```python
from build123d import *

# Parameters (mm, degrees)
F0_R     = 2.4
F1_DEPTH = 3.93
F2_R     = 3.705


with BuildPart() as f1:
    # F0 (on Top) → F1 (new body)
    with BuildSketch(Plane.XY):
        with BuildLine():
            Line((-7.319459, -8.152287), (-7.319459, 4.142713))
            ThreePointArc((-7.319459, 4.142713), (-11.024459, 7.847713), (-14.729459, 4.142713))
            Line((-14.729459, 4.142713), (-14.729459, -15.562287))
            Line((-14.729459, -15.562287), (4.975541, -15.562287))
            ThreePointArc((4.975541, -15.562287), (8.680541, -11.857287), (4.975541, -8.152287))
            Line((4.975541, -8.152287), (-7.319459, -8.152287))
        make_face()
        with BuildLine():
            ThreePointArc((-8.624459, -11.857287), (-8.662221, -12.281351), (-8.774317, -12.69207))
            ThreePointArc((-8.774317, -12.69207), (-8.810969, -12.739379), (-8.868073, -12.757287))
            Line((-8.868073, -12.757287), (-9.624459, -12.757287))
            ThreePointArc((-9.624459, -12.757287), (-9.978012, -12.903734), (-10.124459, -13.257287))
            Line((-10.124459, -13.257287), (-10.124459, -14.013673))
            ThreePointArc((-10.124459, -14.013673), (-10.142367, -14.070777), (-10.189676, -14.107429))
            ThreePointArc((-10.189676, -14.107429), (-11.024459, -14.257287), (-11.859241, -14.107429))
            ThreePointArc((-11.859241, -14.107429), (-11.906551, -14.070777), (-11.924459, -14.013673))
            Line((-11.924459, -14.013673), (-11.924459, -13.257287))
            ThreePointArc((-11.924459, -13.257287), (-12.070905, -12.903734), (-12.424459, -12.757287))
            Line((-12.424459, -12.757287), (-13.180845, -12.757287))
            ThreePointArc((-13.180845, -12.757287), (-13.237949, -12.739379), (-13.274601, -12.69207))
            ThreePointArc((-13.274601, -12.69207), (-13.386697, -12.281351), (-13.424459, -11.857287))
            ThreePointArc((-13.424459, -11.857287), (-13.386697, -11.433224), (-13.274601, -11.022505))
            ThreePointArc((-13.274601, -11.022505), (-13.237949, -10.975195), (-13.180845, -10.957287))
            Line((-13.180845, -10.957287), (-12.424459, -10.957287))
            ThreePointArc((-12.424459, -10.957287), (-12.070905, -10.810841), (-11.924459, -10.457287))
            Line((-11.924459, -10.457287), (-11.924459, -9.700901))
            ThreePointArc((-11.924459, -9.700901), (-11.906551, -9.643797), (-11.859241, -9.607145))
            ThreePointArc((-11.859241, -9.607145), (-11.024459, -9.457287), (-10.189676, -9.607145))
            ThreePointArc((-10.189676, -9.607145), (-10.142367, -9.643797), (-10.124459, -9.700901))
            Line((-10.124459, -9.700901), (-10.124459, -10.457287))
            ThreePointArc((-10.124459, -10.457287), (-9.978012, -10.810841), (-9.624459, -10.957287))
            Line((-9.624459, -10.957287), (-8.868073, -10.957287))
            ThreePointArc((-8.868073, -10.957287), (-8.810969, -10.975195), (-8.774317, -11.022505))
            ThreePointArc((-8.774317, -11.022505), (-8.662221, -11.433224), (-8.624459, -11.857287))
        make_face(mode=Mode.SUBTRACT)
        with Locations((-3.024459, -11.857287)):
            Circle(F0_R, mode=Mode.SUBTRACT)
        with BuildLine():
            ThreePointArc((5.810324, -14.107429), (5.399605, -14.219526), (4.975541, -14.257287))
            ThreePointArc((4.975541, -14.257287), (4.551478, -14.219526), (4.140759, -14.107429))
            ThreePointArc((4.140759, -14.107429), (4.093449, -14.070777), (4.075541, -14.013673))
            Line((4.075541, -14.013673), (4.075541, -13.257287))
            ThreePointArc((4.075541, -13.257287), (3.929095, -12.903734), (3.575541, -12.757287))
            Line((3.575541, -12.757287), (2.819155, -12.757287))
            ThreePointArc((2.819155, -12.757287), (2.762051, -12.739379), (2.725399, -12.69207))
            ThreePointArc((2.725399, -12.69207), (2.575541, -11.857287), (2.725399, -11.022505))
            ThreePointArc((2.725399, -11.022505), (2.762051, -10.975195), (2.819155, -10.957287))
            Line((2.819155, -10.957287), (3.575541, -10.957287))
            ThreePointArc((3.575541, -10.957287), (3.929095, -10.810841), (4.075541, -10.457287))
            Line((4.075541, -10.457287), (4.075541, -9.700901))
            ThreePointArc((4.075541, -9.700901), (4.093449, -9.643797), (4.140759, -9.607145))
            ThreePointArc((4.140759, -9.607145), (4.551478, -9.495049), (4.975541, -9.457287))
            ThreePointArc((4.975541, -9.457287), (5.399605, -9.495049), (5.810324, -9.607145))
            ThreePointArc((5.810324, -9.607145), (5.857633, -9.643797), (5.875541, -9.700901))
            Line((5.875541, -9.700901), (5.875541, -10.457287))
            ThreePointArc((5.875541, -10.457287), (6.021988, -10.810841), (6.375541, -10.957287))
            Line((6.375541, -10.957287), (7.131927, -10.957287))
            ThreePointArc((7.131927, -10.957287), (7.189031, -10.975195), (7.225683, -11.022505))
            ThreePointArc((7.225683, -11.022505), (7.375541, -11.857287), (7.225683, -12.69207))
            ThreePointArc((7.225683, -12.69207), (7.189031, -12.739379), (7.131927, -12.757287))
            Line((7.131927, -12.757287), (6.375541, -12.757287))
            ThreePointArc((6.375541, -12.757287), (6.021988, -12.903734), (5.875541, -13.257287))
            Line((5.875541, -13.257287), (5.875541, -14.013673))
            ThreePointArc((5.875541, -14.013673), (5.857633, -14.070777), (5.810324, -14.107429))
        make_face(mode=Mode.SUBTRACT)
        with Locations((-11.024459, -3.857287)):
            Circle(F0_R, mode=Mode.SUBTRACT)
        with BuildLine():
            ThreePointArc((-12.424459, 5.042713), (-12.070905, 5.189159), (-11.924459, 5.542713))
            Line((-11.924459, 5.542713), (-11.924459, 6.299099))
            ThreePointArc((-11.924459, 6.299099), (-11.906551, 6.356203), (-11.859241, 6.392855))
            ThreePointArc((-11.859241, 6.392855), (-11.024459, 6.542713), (-10.189676, 6.392855))
            ThreePointArc((-10.189676, 6.392855), (-10.142367, 6.356203), (-10.124459, 6.299099))
            Line((-10.124459, 6.299099), (-10.124459, 5.542713))
            ThreePointArc((-10.124459, 5.542713), (-9.978012, 5.189159), (-9.624459, 5.042713))
            Line((-9.624459, 5.042713), (-8.868073, 5.042713))
            ThreePointArc((-8.868073, 5.042713), (-8.810969, 5.024805), (-8.774317, 4.977495))
            ThreePointArc((-8.774317, 4.977495), (-8.662221, 4.566776), (-8.624459, 4.142713))
            ThreePointArc((-8.624459, 4.142713), (-8.662221, 3.718649), (-8.774317, 3.30793))
            ThreePointArc((-8.774317, 3.30793), (-8.810969, 3.260621), (-8.868073, 3.242713))
            Line((-8.868073, 3.242713), (-9.624459, 3.242713))
            ThreePointArc((-9.624459, 3.242713), (-9.978012, 3.096266), (-10.124459, 2.742713))
            Line((-10.124459, 2.742713), (-10.124459, 1.986327))
            ThreePointArc((-10.124459, 1.986327), (-10.142367, 1.929223), (-10.189676, 1.892571))
            ThreePointArc((-10.189676, 1.892571), (-11.024459, 1.742713), (-11.859241, 1.892571))
            ThreePointArc((-11.859241, 1.892571), (-11.906551, 1.929223), (-11.924459, 1.986327))
            Line((-11.924459, 1.986327), (-11.924459, 2.742713))
            ThreePointArc((-11.924459, 2.742713), (-12.070905, 3.096266), (-12.424459, 3.242713))
            Line((-12.424459, 3.242713), (-13.180845, 3.242713))
            ThreePointArc((-13.180845, 3.242713), (-13.237949, 3.260621), (-13.274601, 3.30793))
            ThreePointArc((-13.274601, 3.30793), (-13.386697, 3.718649), (-13.424459, 4.142713))
            ThreePointArc((-13.424459, 4.142713), (-13.386697, 4.566776), (-13.274601, 4.977495))
            ThreePointArc((-13.274601, 4.977495), (-13.237949, 5.024805), (-13.180845, 5.042713))
            Line((-13.180845, 5.042713), (-12.424459, 5.042713))
        make_face(mode=Mode.SUBTRACT)
    extrude(amount=F1_DEPTH)

    # F2
    f2_edges = [f1.edges().sort_by_distance(p)[0] for p in [
        (-14.729459, -15.562287, 1.965),
    ]]
    fillet(f2_edges, radius=F2_R)


solid = f1.part
```
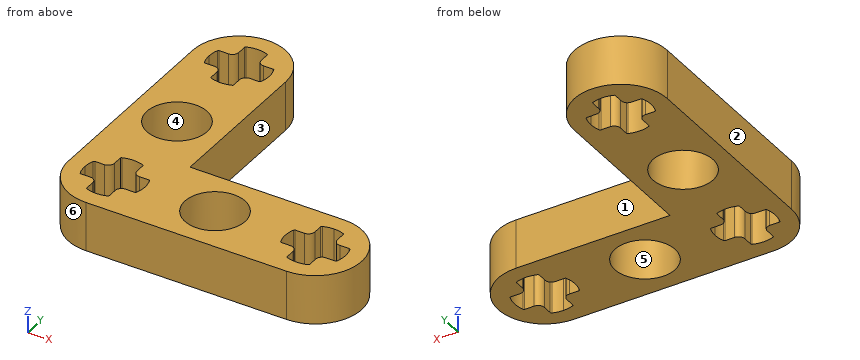
Could you check a few things on this model? Use its own coordinates, in mm. Face numbers are marked on the shaded views. A direction names the side the tool comes from. Round coordinates to 2 decimals unless told otherwise and drop trailing zeros. Loops run counter-clockwise (first coordinate to the right, second up) from the corner with the lowest first, then second, coordinate; pieces in that order, holes last. Notation, with made-up numbers: (19.25, 69) -> (73.25, 69) arc R9 ccw to (73.25, 80) -> close; hole circle Ø6 at (0.5, -10). An arc over 180 degrees is marked (long way). One line per question, with ' | ' between items.
(1) If we section it at C-C on y = -3.5: List the corners of the cut face in (x, z) for me.
Model answer:
outline: (-14.73, 0) -> (-13.4, 0) -> (-13.4, 3.93) -> (-14.73, 3.93) -> close; (-8.65, 0) -> (-7.32, 0) -> (-7.32, 3.93) -> (-8.65, 3.93) -> close
(2) Thinking about a two-plate mould opening in Y: for the marked faces 3, 4, 5 and 6, which applies, released by +Y, released by -Y, zero draft, split by the parting line, or undercut?
Model answer:
face 3: zero draft | face 4: undercut | face 5: undercut | face 6: released by -Y
(3) For the marked faces 1 and 2, which set-ups out of +Z, -Z, +X, -X, +Y, -Y let a thin tool reach every point of the face, with its end or its side?
Model answer:
face 1: +Z, -Z, +X, +Y | face 2: +Z, -Z, -X, +Y, -Y
(4) If we section it at D-D on y = -9: List the corners of the cut face in (x, z) for me.
Model answer:
outline: (-14.73, 0) -> (7.33, 0) -> (7.33, 3.93) -> (-14.73, 3.93) -> close
(5) If we section it at A-A on x = -2.5: List the corners of the cut face in (y, z) for me.
Model answer:
outline: (-15.56, 0) -> (-14.2, 0) -> (-14.2, 3.93) -> (-15.56, 3.93) -> close; (-9.52, 0) -> (-8.15, 0) -> (-8.15, 3.93) -> (-9.52, 3.93) -> close
(6) If we section it at B-B on x = -10.5: List the corners of the cut face in (y, z) for me, and give its area (3 significant figures).
Model answer:
outline: (-15.56, 0) -> (-14.2, 0) -> (-14.2, 3.93) -> (-15.56, 3.93) -> close; (-9.52, 0) -> (-6.2, 0) -> (-6.2, 3.93) -> (-9.52, 3.93) -> close; (-1.52, 0) -> (1.8, 0) -> (1.8, 3.93) -> (-1.52, 3.93) -> close; (6.48, 0) -> (7.81, 0) -> (7.81, 3.93) -> (6.48, 3.93) -> close | area: 36.6 mm^2
(7) For pin 1 Ø1.2 at (x, z) = (0, 3) entering from +Y; pin 2 Ø0.6 at (y, z) = (-10, 1) entering from +X; pin 3 Ø0.8 at (y, z) = (-13.5, 2) entering from +X, each with a flat end and sliding along its axis, tell me the tip position at first contact or that it passes through.
Model answer:
pin 1: stops at y = -8.15 | pin 2: stops at x = 8.34 | pin 3: stops at x = 8.47
(8) If I drill on probe 1 along X at (y, z) = (-13.25, 1.45); probe 2 along X at (y, z) = (-12.5, 0.8); probe 3 along X at (y, z) = (0.25, 0.7), over which ranges is the centre line in solid material (lowest first)?
Model answer:
probe 1: x = -14.46 to -11.92, -10.12 to -4.98, -1.07 to 4.08, 5.88 to 8.41 | probe 2: x = -14.67 to -13.34, -8.71 to -5.34, -0.71 to 2.66, 7.29 to 8.62 | probe 3: x = -14.73 to -7.32
